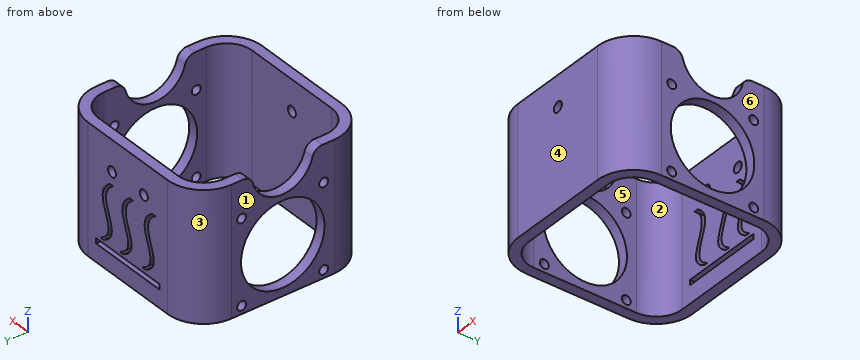
```python
from build123d import *

# Parameters (mm, degrees)
ESTRUSIONE_SOTTILE1_DEPTH = 50
SCHIZZO2_R                = 2
TAGLIO_ESTRUSIONE1_DEPTH  = 10
SCHIZZO3_R                = 12
TAGLIO_ESTRUSIONE2_DEPTH  = 68
RACCORDO1_R               = 4
RACCORDO2_R               = 4
RACCORDO3_R               = 4
RACCORDO4_R               = 4
SCHIZZO4_R                = 2
TAGLIO_ESTRUSIONE3_DEPTH  = 10
SCHIZZO5_W                = 32
SCHIZZO5_H                = 2
TAGLIO_ESTRUSIONE4_DEPTH  = 10
TAGLIO_ESTRUSIONE6_REACH  = 107.925
SCHIZZO8_R                = 16.3
TAGLIO_ESTRUSIONE5_REACH  = 107.925
SCHIZZO7_R                = 1.75


with BuildPart() as part:
    # Schizzo1 → Estrusione-Sottile1 (new body)
    with BuildSketch(Plane.XY):
        with BuildLine():
            Line((-64, -10), (-64, -50))
            ThreePointArc((-64, -50), (-59.899494937, -59.899494937), (-50, -64))
            Line((-50, -64), (-10, -64))
            ThreePointArc((-10, -64), (-0.100505063, -59.899494937), (4, -50))
            Line((4, -50), (4, -10))
            ThreePointArc((4, -10), (-0.100505063, -0.100505063), (-10, 4))
            Line((-10, 4), (-50, 4))
            ThreePointArc((-50, 4), (-59.899494937, -0.100505063), (-64, -10))
        make_face()
        with BuildLine():
            Line((-60, -10), (-60, -50))
            ThreePointArc((-60, -50), (-57.071067812, -57.071067812), (-50, -60))
            Line((-50, -60), (-10, -60))
            ThreePointArc((-10, -60), (-2.928932188, -57.071067812), (0, -50))
            Line((0, -50), (0, -10))
            ThreePointArc((0, -10), (-2.928932188, -2.928932188), (-10, 0))
            Line((-10, 0), (-50, 0))
            ThreePointArc((-50, 0), (-57.071067812, -2.928932188), (-60, -10))
        make_face(mode=Mode.SUBTRACT)
    extrude(amount=ESTRUSIONE_SOTTILE1_DEPTH)

    # Schizzo2 → Taglio-Estrusione1 (cut)
    with BuildSketch(Plane(origin=(0, 4, 0), x_dir=(1, 0, 0), z_dir=(0, 1, 0))):
        with Locations(Location((-38, -38, 0), (0, 0, 180))):
            Circle(SCHIZZO2_R)
        with Locations(Location((-22, -38, 0), (0, 0, 180))):
            Circle(SCHIZZO2_R)
    extrude(amount=-TAGLIO_ESTRUSIONE1_DEPTH, mode=Mode.SUBTRACT)

    # Schizzo3 → Taglio-Estrusione2 (cut)
    with BuildSketch(Plane.ZY.offset(64)):
        with Locations((50, -30)):
            Circle(SCHIZZO3_R)
    extrude(amount=-TAGLIO_ESTRUSIONE2_DEPTH, mode=Mode.SUBTRACT)

    # Raccordo1
    raccordo1_edges = [part.edges().sort_by_distance(p)[0] for p in [
        (-62, -18, 50),
    ]]
    fillet(raccordo1_edges, radius=RACCORDO1_R)

    # Raccordo2
    raccordo2_edges = [part.edges().sort_by_distance(p)[0] for p in [
        (-62, -42, 50),
    ]]
    fillet(raccordo2_edges, radius=RACCORDO2_R)

    # Raccordo3
    raccordo3_edges = [part.edges().sort_by_distance(p)[0] for p in [
        (2, -18, 50),
    ]]
    fillet(raccordo3_edges, radius=RACCORDO3_R)

    # Raccordo4
    raccordo4_edges = [part.edges().sort_by_distance(p)[0] for p in [
        (2, -42, 50),
    ]]
    fillet(raccordo4_edges, radius=RACCORDO4_R)

    # Schizzo4 → Taglio-Estrusione3 (cut)
    with BuildSketch(Plane.XZ.offset(64)):
        with Locations((-30, 38)):
            Circle(SCHIZZO4_R)
    extrude(amount=-TAGLIO_ESTRUSIONE3_DEPTH, mode=Mode.SUBTRACT)

    # Schizzo5 → Taglio-Estrusione4 (cut)
    with BuildSketch(Plane(origin=(0, 4, 0), x_dir=(1, 0, 0), z_dir=(0, 1, 0))):
        with Locations((-30, -7.945849316)):
            Rectangle(SCHIZZO5_W, SCHIZZO5_H)
        with BuildLine():
            Line((-30.960454742, -32.928721256), (-32.639127219, -32.919533938))
            add(Edge.make_bspline(
                [(-27.742758505, -10.323050859), (-39.164938897, -15.912155443), (-21.882006837, -25.659406976), (-32.639127219, -32.919533938)],
                knots=[0, 0, 0, 0, 1, 1, 1, 1], degree=3))
            Line((-27.742758505, -10.323050859), (-26.064086029, -10.332238178))
            add(Edge.make_bspline(
                [(-26.064086029, -10.332238178), (-37.486266421, -15.921342761), (-20.203334361, -25.668594294), (-30.960454742, -32.928721256)],
                knots=[0, 0, 0, 0, 1, 1, 1, 1], degree=3))
        make_face()
        with BuildLine():
            Line((-42.135720019, -33.181656302), (-43.814392495, -33.172468983))
            add(Edge.make_bspline(
                [(-38.918023781, -10.575985905), (-50.340204173, -16.165090488), (-33.057272113, -25.912342021), (-43.814392495, -33.172468983)],
                knots=[0, 0, 0, 0, 1, 1, 1, 1], degree=3))
            Line((-38.918023781, -10.575985905), (-37.239351305, -10.585173223))
            add(Edge.make_bspline(
                [(-37.239351305, -10.585173223), (-48.661531697, -16.174277806), (-31.378599637, -25.921529339), (-42.135720019, -33.181656302)],
                knots=[0, 0, 0, 0, 1, 1, 1, 1], degree=3))
        make_face()
        with BuildLine():
            Line((-21.047266541, -32.963061307), (-22.725939017, -32.953873989))
            add(Edge.make_bspline(
                [(-17.829570303, -10.35739091), (-29.251750695, -15.946495494), (-11.968818635, -25.693747027), (-22.725939017, -32.953873989)],
                knots=[0, 0, 0, 0, 1, 1, 1, 1], degree=3))
            Line((-17.829570303, -10.35739091), (-16.150897827, -10.366578228))
            add(Edge.make_bspline(
                [(-16.150897827, -10.366578228), (-27.573078219, -15.955682812), (-10.290146159, -25.702934345), (-21.047266541, -32.963061307)],
                knots=[0, 0, 0, 0, 1, 1, 1, 1], degree=3))
        make_face()
    extrude(amount=-TAGLIO_ESTRUSIONE4_DEPTH, mode=Mode.SUBTRACT)

    # Taglio-Estrusione6: up to this face of the body (flat: up to its plane)
    taglio_estrusione6_end = Plane(part.part.faces().sort_by_distance((4, -30, 22.393243333))[0])
    # Schizzo8 → Taglio-Estrusione6 (cut, up to the picked face)
    with BuildSketch(Plane.ZY.offset(64), mode=Mode.PRIVATE) as taglio_estrusione6_sk1:
        with Locations(Location((19.401575039, -30.040864416, 0), (0, 0, 270))):
            Circle(SCHIZZO8_R)
    taglio_estrusione6_tool1 = split(extrude(taglio_estrusione6_sk1.sketch, amount=-TAGLIO_ESTRUSIONE6_REACH, mode=Mode.PRIVATE), bisect_by=taglio_estrusione6_end, keep=Keep.BOTH, mode=Mode.PRIVATE)
    add(taglio_estrusione6_tool1.solids().sort_by(Axis((-64, -30.040864, 19.401575), (1, 0, 0)))[0], mode=Mode.SUBTRACT)

    # Taglio-Estrusione5: up to this face of the body (flat: up to its plane)
    taglio_estrusione5_end = Plane(part.part.faces().sort_by_distance((4, -30, 37.359687576))[0])
    # Schizzo7 → Taglio-Estrusione5 (cut, up to the picked face)
    with BuildSketch(Plane.ZY.offset(64), mode=Mode.PRIVATE) as taglio_estrusione5_sk1:
        with Locations(Location((35.701575039, -14, 0), (0, 0, 270))):
            Circle(SCHIZZO7_R)
    taglio_estrusione5_tool1 = split(extrude(taglio_estrusione5_sk1.sketch, amount=-TAGLIO_ESTRUSIONE5_REACH, mode=Mode.PRIVATE), bisect_by=taglio_estrusione5_end, keep=Keep.BOTH, mode=Mode.PRIVATE)
    # Schizzo7 → Taglio-Estrusione5 (cut, up to the picked face)
    with BuildSketch(Plane.ZY.offset(64), mode=Mode.PRIVATE) as taglio_estrusione5_sk2:
        with Locations(Location((35.701575039, -46, 0), (0, 0, 90))):
            Circle(SCHIZZO7_R)
    taglio_estrusione5_tool2 = split(extrude(taglio_estrusione5_sk2.sketch, amount=-TAGLIO_ESTRUSIONE5_REACH, mode=Mode.PRIVATE), bisect_by=taglio_estrusione5_end, keep=Keep.BOTH, mode=Mode.PRIVATE)
    # Schizzo7 → Taglio-Estrusione5 (cut, up to the picked face)
    with BuildSketch(Plane.ZY.offset(64), mode=Mode.PRIVATE) as taglio_estrusione5_sk3:
        with Locations(Location((3.101575039, -46, 0), (0, 0, 270))):
            Circle(SCHIZZO7_R)
    taglio_estrusione5_tool3 = split(extrude(taglio_estrusione5_sk3.sketch, amount=-TAGLIO_ESTRUSIONE5_REACH, mode=Mode.PRIVATE), bisect_by=taglio_estrusione5_end, keep=Keep.BOTH, mode=Mode.PRIVATE)
    # Schizzo7 → Taglio-Estrusione5 (cut, up to the picked face)
    with BuildSketch(Plane.ZY.offset(64), mode=Mode.PRIVATE) as taglio_estrusione5_sk4:
        with Locations(Location((3.101575039, -14, 0), (0, 0, 90))):
            Circle(SCHIZZO7_R)
    taglio_estrusione5_tool4 = split(extrude(taglio_estrusione5_sk4.sketch, amount=-TAGLIO_ESTRUSIONE5_REACH, mode=Mode.PRIVATE), bisect_by=taglio_estrusione5_end, keep=Keep.BOTH, mode=Mode.PRIVATE)
    add(taglio_estrusione5_tool1.solids().sort_by(Axis((-64, -14, 35.701575), (1, 0, 0)))[0], mode=Mode.SUBTRACT)
    add(taglio_estrusione5_tool2.solids().sort_by(Axis((-64, -46, 35.701575), (1, 0, 0)))[0], mode=Mode.SUBTRACT)
    add(taglio_estrusione5_tool3.solids().sort_by(Axis((-64, -46, 3.101575), (1, 0, 0)))[0], mode=Mode.SUBTRACT)
    add(taglio_estrusione5_tool4.solids().sort_by(Axis((-64, -14, 3.101575), (1, 0, 0)))[0], mode=Mode.SUBTRACT)


solid = part.part
```
Can you work these out from the model? Positions are in its coordinate system, mm. Face numbers are marked on the shaded views. A direction names the side the tool comes from. Coordinates: 2 decimals unless noted, no trailing zeros. Order: outer loops, then holes, each group sorted by start corner. A loop starts at its lowest first (then second) coordinate and runs counter-clockwise, first axis right, second up.
1. If we section it at A-A (x = -15): Please give me the cut outline in (y, z).
2. I'm going to push flat-ended pins straight in: pin 1 (4 mm diameter, centred on y = -46, z = 35.7, fed in from -X); pin 2 (3 mm diameter, centred on x = -52.5, z = 31, fed in from +Y); pin 3 (4 mm diameter, centred on x = -55, z = 16.5, fed in from +Y); pin 4 (3 mm diameter, centred on x = -38, z = 38, fed in from +Y). Where does each tip first touch, or does it pass through?
3. I need wall thicknesses on line 1 (X direction, y = -11, z = 27.5); line 2 (Y direction, x = -57.5, z = 16). Which ranges of each line are inside material? Lowest first, please.
4. Thinking about a two-plate mould opening in Y: for the marked faces 3, 4, 5 and 6, which applies, +Y half, -Y half, draft (parallel to the pull), parting line (faces both ways), or undercut?
5. If we section it at B-B (y = -49): Please give me the cut outline in (x, z), then the cut area to 3 significant figures.
6. If we section it at C-C (y = -26): Please give me the cut outline in (x, z).
7. For the marked faces 1 and 2, which set-ups out of +Z, -Z, +X, -X, +Y, -Y let a thin tool reach every point of the face, with its end or its side?
8. If we section it at D-D (x = -1.5): Please give me the cut outline in (y, z), then the cut area to 3 significant figures.
Entries:
1. outline: (-64, 0) - (-60, 0) - (-60, 50) - (-64, 50) - close; (0, 0) - (4, 0) - (4, 6.95) - (0, 6.95) - close; (0, 8.95) - (4, 8.95) - (4, 50) - (0, 50) - close
2. pin 1: stops at x = -64
2. pin 2: stops at y = 3.96
2. pin 3: stops at y = 3.67
2. pin 4: stops at y = -60
3. line 1: x = -64 to -60, 0 to 4
3. line 2: y = -61.82 to -56.61, -3.39 to 1.82
4. face 3: +Y half
4. face 4: -Y half
4. face 5: undercut
4. face 6: draft
5. outline: (-64, 0) - (-60, 0) - (-60, 50) - (-64, 50) - close; (0, 0) - (4, 0) - (4, 50) - (0, 50) - close
5. area: 400 mm2
6. outline: (-64, 0) - (-60, 0) - (-60, 3.61) - (-64, 3.61) - close; (-64, 35.19) - (-60, 35.19) - (-60, 38.69) - (-64, 38.69) - close; (0, 0) - (4, 0) - (4, 3.61) - (0, 3.61) - close; (0, 35.19) - (4, 35.19) - (4, 38.69) - (0, 38.69) - close
7. face 1: +Z, -Z, -X, +Y, -Y
7. face 2: +Z, -Z
8. outline: (-61.12, 0) - (-55.27, 0) - (-55.27, 50) - (-61.12, 50) - close; (-4.73, 0) - (1.12, 0) - (1.12, 50) - (-4.73, 50) - close
8. area: 586 mm2
